Here's how the part is built. I have some questions about the finished solid (model axes, mm). Face numbers are marked on the shaded views. A direction names the side the tool comes from. Round coordinates to 2 decimals unless told otherwise and drop trailing zeros. Order: outer loops, then holes, each group sorted by start corner. A loop starts at its lowest first (then second) coordinate and runs counter-clockwise, first axis right, second up. Notation, with made-up numbers: M 26.25,-17 L 56.25,-17 A35 cw 56.25,19 Z; hole C -27,40 d7. An arc over 180 degrees is marked long. Write each question's results on one line, items separated by ' | '. Start each with the question number.
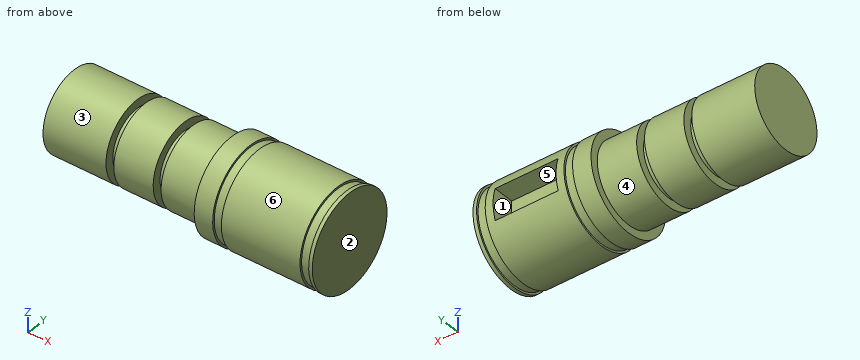
```python
from build123d import *

# Parameters (mm, degrees)
SKETCH1_R           = 6
BOSS_EXTRUDE1_DEPTH = 15
SKETCH2_R           = 5
BOSS_EXTRUDE2_DEPTH = 20
SKETCH3_W           = 8
SKETCH3_H           = 4
CUT_EXTRUDE1_DEPTH  = 3
SKETCH4_W           = 1
SKETCH4_H           = 1.1
SKETCH4_W_2         = 1.1
SKETCH4_H_2         = 0.25


with BuildPart() as part:
    # Sketch1 → Boss-Extrude1 (new body)
    with BuildSketch(Plane(origin=(0, 0, 0), x_dir=(0, 0, -1), z_dir=(1, 0, 0))):
        Circle(SKETCH1_R)
    extrude(amount=BOSS_EXTRUDE1_DEPTH)

    # Sketch2 → Boss-Extrude2 (add)
    with BuildSketch(Plane.ZY):
        Circle(SKETCH2_R)
    extrude(amount=BOSS_EXTRUDE2_DEPTH)

    # Sketch3 → Cut-Extrude1 (cut)
    with BuildSketch(Plane(origin=(0, 6, 0), x_dir=(1, 0, 0), z_dir=(0, 1, 0))):
        with Locations((8.45, 0)):
            Rectangle(SKETCH3_W, SKETCH3_H)
    extrude(amount=-CUT_EXTRUDE1_DEPTH, mode=Mode.SUBTRACT)

    # Sketch4 → Cut-Revolve1 (revolve, cut)
    with BuildSketch(Plane.XY, mode=Mode.PRIVATE) as cut_revolve1_sk:
        with Locations((-5.5, 4.45)):
            Rectangle(SKETCH4_W, SKETCH4_H)
        with Locations((-11.5, 4.45)):
            Rectangle(SKETCH4_W, SKETCH4_H)
        with Locations((2.9, 5.875)):
            Rectangle(SKETCH4_W_2, SKETCH4_H_2)
        with Locations((14, 5.875)):
            Rectangle(SKETCH4_W_2, SKETCH4_H_2)
    revolve(cut_revolve1_sk.sketch.rotate(Axis((0, 0, 0), (-1, 0, 0)), 90), axis=Axis((0, 0, 0), (-1, 0, 0)), mode=Mode.SUBTRACT)


solid = part.part
```
(1) If we mould it in two halves opening along Z, with no side actions, what happens to the marked faces 1, 2 and 3? For each: pulls with the +Z half, pulls with the -Z half, needs draft (parallel to the pull), parting line crosses it, or undercut.
(2) I'm going to push flat-ended pins straight in: pin 1 Ø4 at (x, z) = (-11, 5) entering from -Y; pin 2 Ø1.5 at (x, y) = (-14.5, 4.5) entering from +Z; pin 3 Ø3 at (x, y) = (10, 5) entering from +Z. Where does each tip first touch, or does it pass through?
(3) I want a section at B-B on x = 5.5. Write out the boundary of the cut face in (y, z), and give its area (3 significant figures).
(4) I want a section at C-C on x = -3. Write out the boundary of the cut face in (y, z), and give its area (3 significant figures).
(5) I want a section at A-A on z = -4.5. Give the number of separate pieces and of enclosed holes in the cut face, and give its area (3 significant figures).
(6) On a 3-axis mill with a long thin cutter (end or side, diameter ignored), from which of +Z, -Z, +X, -X, +Y, -Y can I reach the whole of each face in a straight line? I mean the marked faces 4, 5 and 6. Say none if no direction works.
(7) Please list where these lines run through material, in increasing order: line 1 (X direction, y = -5, z = 3.25); line 2 (X direction, y = -4, z = 2); line 3 (X direction, y = -2.5, z = 5).
Solutions:
1) face 1: undercut | face 2: needs draft | face 3: parting line crosses it
2) pin 1: y = -4 | pin 2: z = 3.31 | pin 3: z = 4.87
3) outline: M 3,-2 L 3,2 L 5.66,2 A6 ccw long 5.66,-2 Z | area: 102 mm^2
4) outline: C 0,0 d10 | area: 78.5 mm^2
5) separate pieces: 3 | enclosed holes: 0 | area: 196 mm^2
6) face 4: -X | face 5: +Y | face 6: +X, -X
7) line 1: 0 to 2.35, 3.45 to 13.45, 14.55 to 15 | line 2: -20 to -12, -11 to -6, -5 to 15 | line 3: 0 to 15
